from build123d import *

# Parameters (mm, degrees)
SKETCH1_W           = 33
SKETCH1_H           = 70
BOSS_EXTRUDE1_DEPTH = 20
FILLET1_R           = 0.5
SKETCH2_R           = 0.6
WIRES_2_DEPTH       = 8
SKETCH3_W           = 4.550623551
SKETCH3_H           = 2.528124195
POWER_SWITCH_DEPTH  = 3


with BuildPart() as part:
    # Sketch1 → Boss-Extrude1 (new body)
    with BuildSketch(Plane.XY):
        Rectangle(SKETCH1_W, SKETCH1_H)
    extrude(amount=BOSS_EXTRUDE1_DEPTH)

    # Fillet1
    fillet1_edges = [part.edges().sort_by_distance(p)[0] for p in [
        (-16.5, 0, 20),
        (0, -35, 20),
        (16.5, 0, 20),
        (0, -35, 0),
        (-16.5, 0, 0),
        (0, 35, 0),
        (16.5, 0, 0),
        (16.5, -35, 10),
        (-16.5, -35, 10),
        (-16.5, 35, 10),
        (16.5, 35, 10),
        (0, 35, 20),
    ]]
    fillet(fillet1_edges, radius=FILLET1_R)

    # Sketch2 → Wires 2 (add)
    with BuildSketch(Plane(origin=(0, 35, 0), x_dir=(1, 0, 0), z_dir=(0, 1, 0))):
        with Locations(Location((-14.124921584, -9.591772622, 0), (0, 0, 90))):
            Circle(SKETCH2_R)
        with Locations(Location((-12.864771316, -9.591772622, 0), (0, 0, 90))):
            Circle(SKETCH2_R)
    extrude(amount=WIRES_2_DEPTH)

    # Sketch3 → Power Switch (add)
    with BuildSketch(Plane.XY.offset(20)):
        with Locations((6.042216827, 29.812148032)):
            Rectangle(SKETCH3_W, SKETCH3_H)
    extrude(amount=POWER_SWITCH_DEPTH)


solid = part.part
Build history of the part. All positions in model axes, mm. A direction names the side the tool comes from. Coordinates: 2 decimals unless noted, no trailing zeros. Order: outer loops, then holes, each group sorted by start corner. A loop starts at its lowest first (then second) coordinate and runs counter-clockwise, first axis right, second up. Notation, with made-up numbers: M 32.25,85 L 67.25,85 A23 ccw 67.25,104 Z; hole C 18,3 d7. An arc over 180 degrees is marked long. One line per question, with ' | ' between items. Start each with the question number.
Q1. Saw through at B-B (x = 11). List the corners of the cut face in (y, z), then the cut area to 3 significant figures.
Q2. Flat gauge pins, fed straight in: pin 1 Ø2.5 at (x, z) = (6, 21) entering from +Y; pin 2 Ø12 at (x, z) = (-1.5, 9.5) entering from +Y; pin 3 Ø5 at (x, y) = (1, -13) entering from +Z. Where does each tip first touch, or does it go through?
Q3. 3-axis set-ups, long thin cutter, end or side, ignore diameter. For faces 1 (the face through (8.318, 30, 21)), 2 (the face through (6, 28.548, 21)), 3 (the face through (3.767, 30, 21)), 4 (the face through (6, 31.076, 21)): which of +Z, -Z, +X, -X, +Y, -Y reach the whole face in a straight line?
Q4. Probe L1, parallel to Y at x = -5, z = 16.5; L2, parallel to Z at x = -7, y = 22.5; L3, parallel to X at y = -1.5, z = 19.75. List the from-to ranges inside material, lowest first. Write a range as from..to.
Q5. Saw through at A-A (y = 3). List the corners of the cut face in (x, z), then the cut area to 3 significant figures.
Check values:
1) outline: M -35,0.5 A0.5 ccw -34.5,0 L 34.5,0 A0.5 ccw 35,0.5 L 35,19.5 A0.5 ccw 34.5,20 L -34.5,20 A0.5 ccw -35,19.5 Z | area: 1,400 mm2
2) pin 1: stops at y = 34.93 | pin 2: stops at y = 35 | pin 3: stops at z = 20
3) face 1: +Z, +X, +Y, -Y | face 2: +Z, +X, -X, -Y | face 3: +Z, -X, +Y, -Y | face 4: +Z, +X, -X, +Y
4) L1: y = -35..35 | L2: z = 0..20 | L3: x = -16.43..16.43
5) outline: M -16.5,0.5 A0.5 ccw -16,0 L 16,0 A0.5 ccw 16.5,0.5 L 16.5,19.5 A0.5 ccw 16,20 L -16,20 A0.5 ccw -16.5,19.5 Z | area: 660 mm2
